Part model, mm, in its own coordinate system. Face numbers are marked on the shaded views. A direction names the side the tool comes from. Give positions to 0.01 mm unless a question says otherwise; leave off trailing zeros. Order: outer loops, then holes, each group sorted by start corner. A loop starts at its lowest first (then second) coordinate and runs counter-clockwise, first axis right, second up. Notation, with made-up numbers: M 44.5,-5 L 92.5,-5 A25 ccw 92.5,26 Z; hole C -35.75,12 d9. An arc over 180 degrees is marked long. Answer as a JSON object with one key per item and string values.
from build123d import *

# Parameters (mm, degrees)
SKETCH1_R           = 4
BOSS_EXTRUDE2_DEPTH = 1.5
SKETCH2_W           = 56
SKETCH2_H           = 70
SKETCH2_R           = 2
SKETCH2_R_2         = 5
BOSS_EXTRUDE3_DEPTH = 1.5
FILLET1_R           = 5
FILLET3_R           = 5
FILLET4_R           = 4.5
FILLET5_R           = 3


with BuildPart() as part:
    # Sketch1 → Boss-Extrude2 (new body)
    with BuildSketch(Plane.XY):
        with BuildLine():
            Line((70.488628725, -60.004327551), (95.488628725, -60.004327551))
            ThreePointArc((95.488628725, -60.004327551), (88.442611877, -24.198764926), (88.946986918, 12.290004224))
            ThreePointArc((88.946986918, 12.290004224), (87.020647932, 17.438961897), (81.709367557, 18.857710564))
            ThreePointArc((81.709367557, 18.857710564), (40.759501769, 11.190251314), (-0.573975371, 5.972482924))
            ThreePointArc((-0.573975371, 5.972482924), (-5.927759195, -0.928262318), (1.279261167, -5.862038115))
            ThreePointArc((1.279261167, -5.862038115), (28.82108484, -0.427804063), (56.558651128, 3.897744149))
            ThreePointArc((56.558651128, 3.897744149), (72.640680785, -1.071518566), (79.233271708, -16.559029494))
            ThreePointArc((79.233271708, -16.559029494), (76.676068341, -38.647024387), (70.488628725, -60.004327551))
        make_face()
        Circle(SKETCH1_R, mode=Mode.SUBTRACT)
        with Locations((82.988628725, 12.995672449)):
            Circle(SKETCH1_R, mode=Mode.SUBTRACT)
    extrude(amount=BOSS_EXTRUDE2_DEPTH)

    # Sketch2 → Boss-Extrude3 (add)
    with BuildSketch(Plane.XZ.offset(60.004327551)):
        with Locations((72.308628725, 35)):
            Rectangle(SKETCH2_W, SKETCH2_H)
        with Locations(Location((92.308628725, 42, 0), (0, 0, 270))):
            Circle(SKETCH2_R, mode=Mode.SUBTRACT)
        with Locations(Location((72.308628725, 22, 0), (0, 0, 270))):
            Circle(SKETCH2_R, mode=Mode.SUBTRACT)
        with Locations(Location((52.308628725, 42, 0), (0, 0, 270))):
            Circle(SKETCH2_R, mode=Mode.SUBTRACT)
        with Locations(Location((72.308628725, 62, 0), (0, 0, 270))):
            Circle(SKETCH2_R, mode=Mode.SUBTRACT)
        with Locations(Location((52.308628725, 22, 0), (0, 0, 270))):
            Circle(SKETCH2_R_2, mode=Mode.SUBTRACT)
        with Locations(Location((92.308628725, 22, 0), (0, 0, 270))):
            Circle(SKETCH2_R_2, mode=Mode.SUBTRACT)
        with Locations(Location((92.308628725, 62, 0), (0, 0, 270))):
            Circle(SKETCH2_R_2, mode=Mode.SUBTRACT)
        with Locations(Location((52.308628725, 62, 0), (0, 0, 270))):
            Circle(SKETCH2_R_2, mode=Mode.SUBTRACT)
    extrude(amount=BOSS_EXTRUDE3_DEPTH)

    # Fillet1
    fillet1_edges = [part.edges().sort_by_distance(p)[0] for p in [
        (100.308628725, -60.754327551, 0),
        (100.308628725, -60.754327551, 70),
        (44.308628725, -60.754327551, 70),
        (44.308628725, -60.754327551, 0),
    ]]
    fillet(fillet1_edges, radius=FILLET1_R)

    # Fillet3
    fillet3_edges = [part.edges().sort_by_distance(p)[0] for p in [
        (70.488628725, -60.004327551, 0.75),
    ]]
    fillet(fillet3_edges, radius=FILLET3_R)

    # Fillet4
    fillet4_edges = [part.edges().sort_by_distance(p)[0] for p in [
        (95.488628725, -60.004327551, 0.751620525),
    ]]
    fillet(fillet4_edges, radius=FILLET4_R)

    # Fillet5
    fillet5_edges = [part.edges().sort_by_distance(p)[0] for p in [
        (82.922685412, -60.004327551, 1.5),
    ]]
    fillet(fillet5_edges, radius=FILLET5_R)


solid = part.part
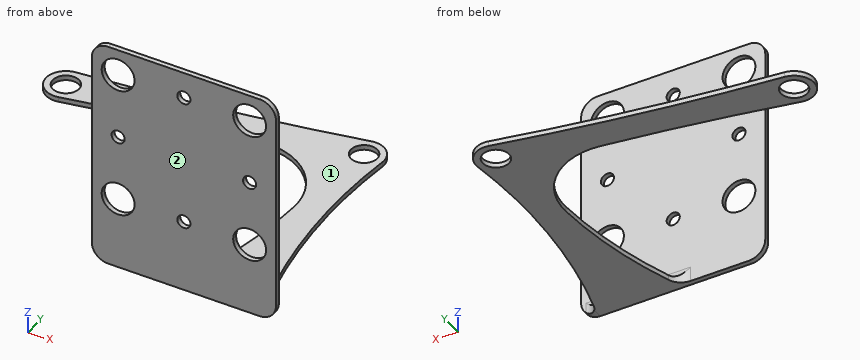
1. Which spindle directions (+Z, -Z, +X, -X, +Y, -Y) get a long thin tool onto all of the face, cutting with end or side? Do the marked faces 1 and 2. Say none if no direction does.
Worked answers:
{"face 1": "+Z, +X, -X, +Y", "face 2": "+Z, -Z, +X, -X, -Y"}
2. Probe line 1 along X through (y, z) = (-60.55, 42); line 2 along X through (y, z) = (-60.95, 22); line 3 along Y through (x, z) = (58.5, 58). List the from-to ranges inside material, lowest first.
Worked answers:
{"line 1": "x = 44.31 to 50.31, 54.31 to 90.31, 94.31 to 100.31", "line 2": "x = 44.31 to 47.31, 57.31 to 70.31, 74.31 to 87.31, 97.31 to 100.31", "line 3": "y = -61.5 to -60"}
3. Pin check, flat tips, straight feed: P1, Ø13, axis at x = 92.31, z = 62, coming from the +Y side; P2, Ø6, axis at x = 92.31, z = 22, coming from the -Y side; P3, Ø1.2, axis at y = -61, z = 24.5, coming from the -X side. Stop position of each tip, or through.
Worked answers:
{"P1": "stops at y = -60", "P2": "passes through", "P3": "stops at x = 44.31"}
4. Cut at D-D on y = -35. Give the cut face in (x, z), plus the area to 3 significant figures.
Worked answers:
{"outline": "M 77.36,0 L 89.76,0 L 89.76,1.5 L 77.36,1.5 Z", "area": "18.6 mm^2"}
5. Cut at A-A on z = 42. Give the cut face in (x, y), plus the area to 3 significant figures.
Worked answers:
{"outline": "M 44.31,-61.5 L 50.31,-61.5 L 50.31,-60 L 44.31,-60 Z; M 54.31,-61.5 L 90.31,-61.5 L 90.31,-60 L 54.31,-60 Z; M 94.31,-61.5 L 100.31,-61.5 L 100.31,-60 L 94.31,-60 Z", "area": "72.0 mm^2"}
6. Cut at C-C on z = 22. Give the cut face in (x, y).
Worked answers:
{"outline": "M 44.31,-61.5 L 47.31,-61.5 L 47.31,-60 L 44.31,-60 Z; M 57.31,-61.5 L 70.31,-61.5 L 70.31,-60 L 57.31,-60 Z; M 74.31,-61.5 L 87.31,-61.5 L 87.31,-60 L 74.31,-60 Z; M 97.31,-61.5 L 100.31,-61.5 L 100.31,-60 L 97.31,-60 Z"}
7. Cut at B-B on y = 0. Give the cut face in (x, z).
Worked answers:
{"outline": "M -6,0 L -4,0 L -4,1.5 L -6,1.5 Z; M 4,0 L 31.27,0 L 31.27,1.5 L 4,1.5 Z; M 71.35,0 L 87.93,0 L 87.93,1.5 L 71.35,1.5 Z"}
